from build123d import *

# Parameters (mm, degrees)
EXTRUDE_1_DEPTH = 2
FILLET_1_R      = 4
FILLET_2_R      = 1


with BuildPart() as part:
    # Эскиз1 → Бобышка-Вытянуть1 (new body)
    with BuildSketch(Plane.XY):
        Polygon((0, 0), (29, 7.770526581), (29, 23.299669287), (0, 15.529142706), align=None)
    extrude(amount=EXTRUDE_1_DEPTH)

    # Скругление1
    fillet_1_edges = [part.edges().sort_by_distance(p)[0] for p in [
        (0, 15.529142706, 1),
        (29, 23.299669287, 1),
        (29, 7.770526581, 1),
        (0, 0, 1),
    ]]
    fillet(fillet_1_edges, radius=FILLET_1_R)

    # Скругление2
    fillet_2_edges = [part.edges().sort_by_distance(p)[0] for p in [
        (0, 8.836368123, 2),
        (13.46472382, 19.13700458, 2),
        (15.53527618, 4.162664707, 2),
        (29, 14.463301164, 2),
        (27.435045716, 21.260181156, 2),
        (28.173413361, 8.404788816, 2),
        (1.564954284, 2.03948813, 2),
        (0.826586639, 14.89488047, 2),
    ]]
    fillet(fillet_2_edges, radius=FILLET_2_R)


solid = part.part
Check sheet for the modelled part. Datum: model origin and axes. Units: mm. Round coordinates to 2 decimals unless told otherwise and drop trailing zeros. Order: outer loops, then holes, each group sorted by start corner. A loop starts at its lowest first (then second) coordinate and runs counter-clockwise, first axis right, second up. Notation, with made-up numbers: M 46,-2 L 71,-2 A37 cw 71,36 Z; hole C 44,14.25 d2. An arc over 180 degrees is marked long. One line per item, written item: value. Start each with the question number.
1. Gauge pin test, flat end, axial feed: P1, Ø1, axis at x = 12.5, z = 1.5, coming from the +Y side. Record the tip position at first contact, or that the pin passes through.
2. Section check A-A on z = 0.6. Enter the section's corners in (x, y), and give its area (3 significant figures).
3. Scan lines: line 1 along Y through (x, z) = (3, 1.1); line 2 along Z through (x, y) = (11.5, 4); line 3 along Z through (x, y) = (14.75, 4.5). Record each from-to range of solid material in increasing order.
Results found:
1. P1: y = 18.96
2. outline: M 0,5.21 A4 ccw 5.04,1.35 L 26.04,6.98 A4 ccw 29,10.84 L 29,18.09 A4 ccw 23.96,21.95 L 2.96,16.32 A4 ccw 0,12.46 Z
2. area: 434 mm^2
3. line 1: 1.35 to 16.33
3. line 2: 0 to 1.99
3. line 3: 0 to 1.88
